Input: part model. Units: mm. Frame: model coordinates. Face numbers are marked on the shaded views. A direction names the side the tool comes from. Coordinates: 2 decimals unless noted, no trailing zeros. Answer as a JSON object with one key per item and string values. Group by question number.
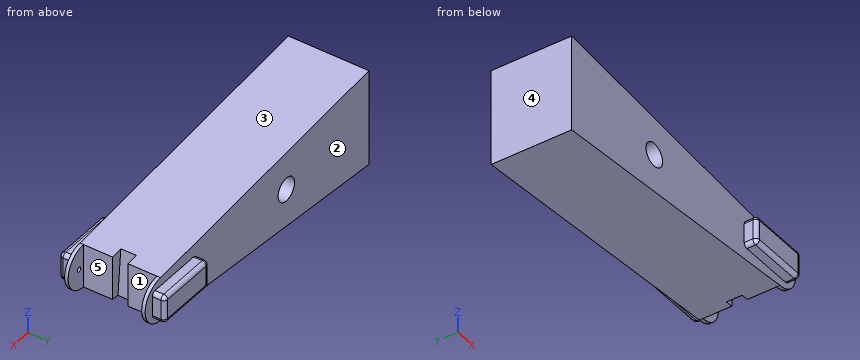
from build123d import *

# Parameters (mm, degrees)
BOSS_EXTRUDE1_DEPTH  = 103
FILLET1_R            = 0.001
SKETCH3_W            = 80
SKETCH3_H            = 35
BOSS_EXTRUDE2_DEPTH  = 16
FILLET2_R            = 5
SKETCH4_R            = 15
CUT_EXTRUDE1_DEPTH   = 424.88163248
CUT_EXTRUDE10_DEPTH  = 47
SKETCH17_W           = 20
SKETCH17_H           = 20
CUT_EXTRUDE13_DEPTH  = 94
FILLET2_OF_MIRROR1_R = 5
SKETCH19_R           = 3
CUT_EXTRUDE14_DEPTH  = 10
CUT_EXTRUDE15_START  = -10
SKETCH20_R           = 3
CUT_EXTRUDE15_DEPTH  = 10


with BuildPart() as part:
    # Sketch1 → Boss-Extrude1 (new body)
    with BuildSketch(Plane(origin=(0, 0, 0), x_dir=(1, 0, 0), z_dir=(0, 1, 0))):
        with BuildLine():
            Line((0, -62), (0, 62))
            Line((0, 62), (378.47589091, 28))
            ThreePointArc((378.47589091, 28), (406.47589091, 0), (378.47589091, -28))
            Line((378.47589091, -28), (0, -62))
        make_face()
    extrude(amount=BOSS_EXTRUDE1_DEPTH)

    # Fillet1
    fillet1_edges = [part.edges().sort_by_distance(p)[0] for p in [
        (378.47589091, 51.5, 28),
        (406.47589091, 103, 0),
        (378.47589091, 51.5, -28),
        (406.47589091, 0, 0),
        (0, 51.5, -62),
        (0, 103, 0),
        (0, 51.5, 62),
        (0, 0, 0),
        (189.237945455, 0, 45),
        (189.237945455, 0, -45),
        (189.237945455, 103, 45),
        (189.237945455, 103, -45),
    ]]
    fillet(fillet1_edges, radius=FILLET1_R)

    # Sketch3 → Boss-Extrude2 (add)
    with BuildSketch(Plane(origin=(0, 0, 0), x_dir=(-1, 0, 0), z_dir=(0, -1, 0))):
        with Locations((-353.47589091, 0)):
            Rectangle(SKETCH3_W, SKETCH3_H)
    boss_extrude2 = extrude(amount=BOSS_EXTRUDE2_DEPTH)

    # Fillet2
    fillet2_edges = [part.edges().sort_by_distance(p)[0] for p in [
        (313.47589091, -8, 17.5),
        (313.47589091, -8, -17.5),
        (393.47589091, -8, -17.5),
        (393.47589091, -8, 17.5),
        (313.47589091, -16, 0),
        (353.47589091, -16, -17.5),
        (393.47589091, -16, 0),
        (353.47589091, -16, 17.5),
    ]]
    fillet(fillet2_edges, radius=FILLET2_R)

    # Sketch4 → Cut-Extrude1 (cut, through all)
    with BuildSketch(Plane.XZ):
        with Locations(Location((150.001, 0, 0), (0, 0, 270))):
            Circle(SKETCH4_R)
    extrude(amount=-CUT_EXTRUDE1_DEPTH, mode=Mode.SUBTRACT)

    # Sketch15 → Cut-Extrude10 (cut, symmetric)
    with BuildSketch(Plane(origin=(0, 51.5, 0), x_dir=(-1, 0, 0), z_dir=(0, -1, 0))):
        with BuildLine():
            Line((-378.47589091, 29), (-378.47589091, -29))
            ThreePointArc((-378.47589091, -29), (-407.47589091, 0), (-378.47589091, 29))
        make_face()
    extrude(amount=CUT_EXTRUDE10_DEPTH, both=True, mode=Mode.SUBTRACT)

    # Sketch17 → Cut-Extrude13 (cut)
    with BuildSketch(Plane(origin=(5.525118961, 0, -61.50365651), x_dir=(-0.9959891866048521, 0, -0.08947368421052682), z_dir=(0.08947368421052682, 0, -0.9959891866048521))):
        with Locations((-374.452586753, 51.5)):
            Rectangle(SKETCH17_W, SKETCH17_H)
    extrude(amount=-CUT_EXTRUDE13_DEPTH, mode=Mode.SUBTRACT)

    # Mirror1: Boss-Extrude2 across plane
    add(boss_extrude2.mirror(Plane(origin=(0, 51.5, 0), x_dir=(0, 0, 1), z_dir=(0, -1, 0))))

    # Fillet2 of Mirror1
    fillet2_of_mirror1_edges = [part.edges().sort_by_distance(p)[0] for p in [
        (313.47589091, 111, 17.5),
        (313.47589091, 111, -17.5),
        (393.47589091, 111, -17.5),
        (393.47589091, 111, 17.5),
        (313.47589091, 119, 0),
        (353.47589091, 119, -17.5),
        (393.47589091, 119, 0),
        (353.47589091, 119, 17.5),
    ]]
    fillet(fillet2_of_mirror1_edges, radius=FILLET2_OF_MIRROR1_R)

    # Sketch19 → Cut-Extrude14 (cut)
    with BuildSketch(Plane(origin=(0, 4.5, 0), x_dir=(1, 0, 0), z_dir=(0, 1, 0))):
        with Locations(Location((386.47589091, 0, 0), (0, 0, 270))):
            Circle(SKETCH19_R)
    extrude(amount=-CUT_EXTRUDE14_DEPTH, mode=Mode.SUBTRACT)

    # Sketch20 → Cut-Extrude15 (cut)
    with BuildSketch(Plane.XZ.offset(-98.5).offset(CUT_EXTRUDE15_START)):
        with Locations(Location((386.47589091, 0, 0), (0, 0, 90))):
            Circle(SKETCH20_R)
    extrude(amount=CUT_EXTRUDE15_DEPTH, mode=Mode.SUBTRACT)


solid = part.part
Q1. Access query for the marked faces 4 and 5. Directions: +Z, -Z, +X, -X, +Y, -Y. A direction counts if a zero-diameter tool reaches every point of the face in a straight line with its end or side. Return the directions, or none.
Q2. Pin query (flat end, axial travel): pin 1 Ø12 at (x, z) = (371.5, -13) entering from -Y; pin 2 Ø12 at (y, z) = (-7, 2) entering from +X; pin 3 Ø11 at (y, z) = (75, 7.5) entering from +X; pin 4 Ø10 at (x, z) = (44, 22) entering from -Y. Return the tip coordinate at first contact, or that it passes through.
Q3. Draft query along Y for the marked faces 1, 2 and 3. Return one class per face: released by +Y, released by -Y, zero draft, split by the parting line, or undercut.
Q4. Line query: line 1 (X direction, y = 1.25, z = 0); line 2 (X direction, y = 41, z = 0); line 3 (Y direction, x = 23.5, z = -47). Output: solid intervals per line, ascending. Write a range as from..to.
Filled in:
{
 "1": {"face 4": "+Z, -Z, -X, +Y, -Y", "face 5": "+Z, -Z, +X"},
 "2": {"pin 1": "y = -16", "pin 2": "x = 393.48", "pin 3": "x = 378.48", "pin 4": "y = 0"},
 "3": {"face 1": "undercut", "face 2": "released by +Y", "face 3": "zero draft"},
 "4": {"line 1": "0..135, 165..383.48, 389.48..406.48", "line 2": "0..135, 165..378.48", "line 3": "0..103"}
}
